Geometry: final body of the model. Coordinates: model frame, mm. A direction names the side the tool comes from. Give positions to 0.01 mm unless a question says otherwise; leave off trailing zeros. Write each loop counter-clockwise with the first axis right and the second up, starting at its lowest first coordinate (ties: lowest second). Pieces come first, ordered by that corner, then holes.
```python
from build123d import *

# Parameters (mm, degrees)
SKETCH_1_W           = 36
SKETCH_1_H           = 20
EXTRUDE_1_DEPTH      = 32.5
SKETCH_4_R           = 5
CUT_EXTRUDE_2_DEPTH  = 47
SKETCH_9_R           = 2.25
CUT_EXTRUDE_7_DEPTH  = 27
SKETCH_10_W          = 11
SKETCH_10_H          = 6
EXTRUDE_2_DEPTH      = 4
SKETCH_11_R          = 2.25
CUT_EXTRUDE_8_DEPTH  = 20
SKETCH_12_R          = 4.3
CUT_EXTRUDE_9_DEPTH  = 5
SKETCH_13_W          = 7.5
SKETCH_13_H          = 4
CUT_EXTRUDE_10_DEPTH = 22
SKETCH_14_R          = 4.3
CUT_EXTRUDE_11_DEPTH = 7
FILLET_1_R           = 7


with BuildPart() as part:
    # Эскиз1 → Бобышка-Вытянуть1 (new body)
    with BuildSketch(Plane(origin=(0, 0, 0), x_dir=(1, 0, 0), z_dir=(0, 1, 0))):
        with Locations((18, 10)):
            Rectangle(SKETCH_1_W, SKETCH_1_H)
    extrude(amount=EXTRUDE_1_DEPTH)

    # Эскиз4 → Вырез-Вытянуть2 (cut)
    with BuildSketch(Plane.XY):
        with Locations((18, 25.5)):
            Circle(SKETCH_4_R)
        with BuildLine():
            ThreePointArc((13.056570017, 24.75), (13, 25.5), (13.056570017, 26.25))
            Line((13.056570017, 26.25), (0, 26.25))
            Line((0, 26.25), (0, 24.75))
            Line((0, 24.75), (13.056570017, 24.75))
        make_face()
    extrude(amount=-CUT_EXTRUDE_2_DEPTH, mode=Mode.SUBTRACT)

    # Эскиз9 → Вырез-Вытянуть7 (cut)
    with BuildSketch(Plane.XY):
        with Locations((30.5, 9)):
            Circle(SKETCH_9_R)
        with Locations((5.5, 9)):
            Circle(SKETCH_9_R)
    extrude(amount=-CUT_EXTRUDE_7_DEPTH, mode=Mode.SUBTRACT)

    # Эскиз10 → Бобышка-Вытянуть2 (add)
    with BuildSketch(Plane.XY):
        with Locations((18, 9)):
            Rectangle(SKETCH_10_W, SKETCH_10_H)
    extrude(amount=EXTRUDE_2_DEPTH)

    # Эскиз11 → Вырез-Вытянуть8 (cut)
    with BuildSketch(Plane(origin=(0, 32.5, 0), x_dir=(1, 0, 0), z_dir=(0, 1, 0))):
        with Locations(Location((5, 10, 0), (0, 0, 270))):
            Circle(SKETCH_11_R)
    extrude(amount=-CUT_EXTRUDE_8_DEPTH, mode=Mode.SUBTRACT)

    # Эскиз12 → Вырез-Вытянуть9 (cut)
    with BuildSketch(Plane(origin=(0, 32.5, 0), x_dir=(1, 0, 0), z_dir=(0, 1, 0))):
        with Locations(Location((5, 10, 0), (0, 0, 270))):
            Circle(SKETCH_12_R)
    extrude(amount=-CUT_EXTRUDE_9_DEPTH, mode=Mode.SUBTRACT)

    # Эскиз13 → Вырез-Вытянуть10 (cut)
    with BuildSketch(Plane(origin=(0, 0, -20), x_dir=(-1, 0, 0), z_dir=(0, 0, -1))):
        with Locations((-5, 18.75)):
            Rectangle(SKETCH_13_W, SKETCH_13_H)
    extrude(amount=-CUT_EXTRUDE_10_DEPTH, mode=Mode.SUBTRACT)

    # Эскиз14 → Вырез-Вытянуть11 (cut)
    with BuildSketch(Plane(origin=(0, 0, -20), x_dir=(-1, 0, 0), z_dir=(0, 0, -1))):
        with Locations((-30.5, 9)):
            Circle(SKETCH_14_R)
        with Locations((-5.5, 9)):
            Circle(SKETCH_14_R)
    extrude(amount=-CUT_EXTRUDE_11_DEPTH, mode=Mode.SUBTRACT)

    # Скругление1
    # the kernel refuses this fillet: 7 mm, written as the material it takes off along each edge
    with BuildSketch(Plane(origin=(36, 32.5, 17.5), x_dir=(0, -1, 0), z_dir=(0, 0, -1))) as fillet_1_piece_1:
        with BuildLine():
            CenterArc((FILLET_1_R, FILLET_1_R), FILLET_1_R, 180, 90)
            Line((0, FILLET_1_R), (0, 0))
            Line((0, 0), (FILLET_1_R, 0))
        make_face()
    extrude(amount=55, mode=Mode.SUBTRACT)
    with BuildSketch(Plane(origin=(0, 32.5, -37.399263634), x_dir=(1, 0, 0), z_dir=(0, 0, 1))) as fillet_1_piece_2:
        with BuildLine():
            CenterArc((6.959705454, -7), FILLET_1_R, 90, 83.849360172)
            Line((0, -6.25), (0, 0))
            Line((0, 0), (6.959705454, 0))
        make_face()
    extrude(amount=54.798527268, mode=Mode.SUBTRACT)


solid = part.part
```
Item 1: Section B-B, the plane x = 10.5. Return the cut outline in (y, z).
Found:
outline: (0, -20) - (24.75, -20) - (24.75, 0) - (0, 0) - close; (26.25, -20) - (32.5, -20) - (32.5, 0) - (26.25, 0) - close
Item 2: Section D-D, the plane z = -16.75. Return the cut outline in (x, y).
Found:
outline: (0, 0) - (36, 0) - (36, 25.5) arc R7 ccw to (29, 32.5) - (6.96, 32.5) arc R7 ccw to (0, 26.25) - (13.06, 26.25) arc R5 cw (long way) to (13.06, 24.75) - (0, 24.75) - close; hole circle Ø8.6 at (5.5, 9); hole (1.25, 16.75) - (8.75, 16.75) - (8.75, 20.75) - (1.25, 20.75) - close; hole circle Ø8.6 at (30.5, 9)
Item 3: Pin query (flat end, axial travel): pin 1 Ø8 at (x, y) = (9, 20.5) entering from +Z; pin 2 Ø1.2 at (x, z) = (16, 2) entering from -Y; pin 3 Ø1.2 at (y, z) = (8.5, 2) entering from +X; pin 4 Ø8 at (x, y) = (18, 25.5) entering from -Z. Return the tip coordinate at first contact, or that it passes through.
Found:
pin 1: stops at z = 0
pin 2: stops at y = 6
pin 3: stops at x = 23.5
pin 4: passes through
Item 4: Section C-C, the plane z = -10.25. State how many separate pieces and enclosed holes the cut face has, plus the area to 3 significant figures.
Found:
separate pieces: 2
enclosed holes: 2
area: 911 mm2
Item 5: Section A-A, the plane y = 9. Return the cut outline in (x, z), plus the area to 3 significant figures.
Found:
outline: (0, -20) - (1.2, -20) - (1.2, -13) - (3.25, -13) - (3.25, 0) - (0, 0) - close; (7.75, -13) - (9.8, -13) - (9.8, -20) - (26.2, -20) - (26.2, -13) - (28.25, -13) - (28.25, 0) - (23.5, 0) - (23.5, 4) - (12.5, 4) - (12.5, 0) - (7.75, 0) - close; (32.75, -13) - (34.8, -13) - (34.8, -20) - (36, -20) - (36, 0) - (32.75, 0) - close
area: 527 mm2
Item 6: Reachability of faces 4 (the face through (5.099, 14.655, -12.248)), 5 (the face through (5.1, 16.75, -12.4)), 6 (the face through (26.4, 10.3, -16.5)) from +Z, -Z, +X, -X, +Y, -Y: full face, straight path, thin tool, end or side. Return the list, or none.
Found:
face 4: +Y
face 5: +Z, -Z
face 6: -Z
Item 7: Line query: L1, parallel to X at y = 27.1, z = -10; L2, parallel to Y at x = 12, z = -9; L3, parallel to X at y = 22.5, z = -11. Output: solid intervals per line, ascending.
Found:
L1: x = 0.15 to 2.75, 7.25 to 13.26, 22.74 to 35.81
L2: y = 0 to 24.75, 26.25 to 32.5
L3: x = 0 to 2.98, 7.02 to 14, 22 to 36
Item 8: Pull-direction query (Z, two-part tool) for faces 1 (the face through (4, 7, -13)), 2 (the face through (5.099, 22.778, -12.248)), 3 (the face through (36, 13, -10)); classes: +Z half, -Z half, draft (parallel to the pull), parting line (faces both ways), or undercut.
Found:
face 1: -Z half
face 2: undercut
face 3: draft
